Could you check a few things on this model? Use its own coordinates, in mm. Face numbers are marked on the shaded views. A direction names the side the tool comes from. Give positions to 0.01 mm unless a question says otherwise; leave off trailing zeros. Write each loop counter-clockwise with the first axis right and the second up, starting at its lowest first coordinate (ties: lowest second). Pieces come first, ordered by that corner, then holes. Notation, with made-up numbers: (60, -39) - (103, -39) arc R13 cw to (103, -30) - close; hole circle Ø3 at (72.25, 76). An arc over 180 degrees is marked (long way). Answer in a Markdown table with one row per item.
Autodesk Inventor part; units mm, degrees
ref_plane "YZ Plane" through (0, 0, 0) normal (1, 0, 0) x (0, 1, 0)
ref_plane "XZ Plane" through (0, 0, 0) normal (0, 1, 0) x (-1, 0, 0)
ref_plane "XY Plane" through (0, 0, 0) normal (0, 0, 1) x (1, 0, 0)
sketch "スケッチ1" plane through (0, 0, 0) normal (0, 0, 1) x (1, 0, 0)
  circle A0 centre (5, 5) radius 1.55
  circle A1 centre (5, -5) radius 1.55
  line L0 (0, 0) -> (60, 0) construction
  circle A2 centre (60, 0) radius 1.55
  line L1 (0, 10) -> (0, -10)
  line L2 (0, -10) -> (10, -10)
  line L3 (10, -10) -> (60.4762, -5.9811)
  line L4 (10, 10) -> (60.4762, 5.9811)
  arc A3 (60.4762, -5.9811) -> (60.4762, 5.9811) centre (60, 0) ccw
  line L5 (55.0583, -3.4029) -> (11, -6.9109)
  line L6 (55.0583, 3.4029) -> (11, 6.9109)
  arc A4 (55.0583, 3.4029) -> (55.0583, -3.4029) centre (60, 0) ccw
  line L7 (11, -6.9109) -> (11, 6.9109)
  line L8 (5, -5) -> (5, 5) construction
  line L9 (0, 10) -> (10, 10)
  line L10 (8.01, 6.7378) -> (8.01, 3.2622) construction
  line L11 (8.01, 3.2622) -> (5, 1.5244) construction
  line L12 (5, 1.5244) -> (1.99, 3.2622) construction
  line L13 (1.99, 3.2622) -> (1.99, 6.7378) construction
  line L14 (1.99, 6.7378) -> (5, 8.4756) construction
  line L15 (5, 8.4756) -> (8.01, 6.7378) construction
  arc A5 (4.0907, 2.0494) -> (5.9093, 2.0494) centre (5, 2.5744) ccw construction
  arc A6 (7.1007, 2.7372) -> (8.01, 4.3122) centre (7.1007, 3.7872) ccw construction
  arc A7 (8.01, 5.6878) -> (7.1007, 7.2628) centre (7.1007, 6.2128) ccw construction
  arc A8 (5.9093, 7.9506) -> (4.0907, 7.9506) centre (5, 7.4256) ccw construction
  arc A9 (2.8993, 7.2628) -> (1.99, 5.6878) centre (2.8993, 6.2128) ccw construction
  arc A10 (1.99, 4.3122) -> (2.8993, 2.7372) centre (2.8993, 3.7872) ccw construction
  line L16 (8.01, -6.7378) -> (8.01, -3.2622) construction
  line L17 (8.01, -3.2622) -> (5, -1.5244) construction
  line L18 (5, -1.5244) -> (1.99, -3.2622) construction
  line L19 (1.99, -3.2622) -> (1.99, -6.7378) construction
  line L20 (1.99, -6.7378) -> (5, -8.4756) construction
  line L21 (5, -8.4756) -> (8.01, -6.7378) construction
  arc A11 (5.9093, -2.0494) -> (4.0907, -2.0494) centre (5, -2.5744) ccw construction
  arc A12 (8.01, -4.3122) -> (7.1007, -2.7372) centre (7.1007, -3.7872) ccw construction
  arc A13 (7.1007, -7.2628) -> (8.01, -5.6878) centre (7.1007, -6.2128) ccw construction
  arc A14 (4.0907, -7.9506) -> (5.9093, -7.9506) centre (5, -7.4256) ccw construction
  arc A15 (1.99, -5.6878) -> (2.8993, -7.2628) centre (2.8993, -6.2128) ccw construction
  arc A16 (2.8993, -2.7372) -> (1.99, -4.3122) centre (2.8993, -3.7872) ccw construction
  circle A17 centre (60, 0) radius 1.55
  line L22 (63.51, 2.0265) -> (63.51, -2.0265)
  line L23 (63.51, -2.0265) -> (60, -4.053)
  line L24 (60, -4.053) -> (56.49, -2.0265)
  line L25 (56.49, -2.0265) -> (56.49, 2.0265)
  line L26 (56.49, 2.0265) -> (60, 4.053)
  line L27 (60, 4.053) -> (63.51, 2.0265)
  arc A18 (59.0907, -3.528) -> (60.9093, -3.528) centre (60, -3.003) ccw
  arc A19 (62.6007, -2.5515) -> (63.51, -0.9765) centre (62.6007, -1.5015) ccw
  arc A20 (63.51, 0.9765) -> (62.6007, 2.5515) centre (62.6007, 1.5015) ccw
  arc A21 (60.9093, 3.528) -> (59.0907, 3.528) centre (60, 3.003) ccw
  arc A22 (57.3993, 2.5515) -> (56.49, 0.9765) centre (57.3993, 1.5015) ccw
  arc A23 (56.49, -0.9765) -> (57.3993, -2.5515) centre (57.3993, -1.5015) ccw
  line L28 (60, 4.053) -> (60, -4.053) construction
  circle A24 centre (5, 5) radius 3.005
  circle A25 centre (5, -5) radius 3.005
  point P0 (5, 0)
  point P1 (8.01, 3.2622)
  point P2 (8.01, 6.7378)
  point P3 (5, 8.4756)
  point P4 (1.99, 6.7378)
  point P5 (2.8993, 2.7372)
  point P6 (1.99, 4.3122)
  point P7 (1.99, 5.6878)
  point P8 (2.8993, 7.2628)
  point P9 (4.0907, 7.9506)
  point P10 (5.9093, 7.9506)
  point P11 (7.1007, 7.2628)
  point P12 (8.01, 5.6878)
  point P13 (8.01, 4.3122)
  point P14 (7.1007, 2.7372)
  point P15 (7.1007, -2.7372)
  point P16 (8.01, -4.3122)
  point P17 (8.01, -5.6878)
  point P18 (7.1007, -7.2628)
  point P19 (5.9093, -7.9506)
  point P20 (4.0907, -7.9506)
  point P21 (2.8993, -7.2628)
  point P22 (1.99, -5.6878)
  point P23 (1.99, -4.3122)
  point P24 (2.8993, -2.7372)
  point P25 (1.99, -6.7378)
  point P26 (5, -8.4756)
  point P27 (56.49, 2.0265)
  point P28 (56.49, -2.0265)
  point P29 (62.6007, -2.5515)
  point P30 (57.3993, -2.5515)
  point P31 (56.49, -0.9765)
  point P32 (56.49, 0.9765)
  point P33 (57.3993, 2.5515)
  point P34 (59.0907, 3.528)
  point P35 (60.9093, 3.528)
  point P36 (62.6007, 2.5515)
  point P37 (63.51, 0.9765)
  point P38 (63.51, -0.9765)
  dimension "d0" = 10
  dimension "d1" = 3.1
  dimension "d2" = 3.1
  dimension "d3" = 60
  dimension "d4" = 6
  dimension "d33" = 3
  dimension "d34" = 6
  dimension "d35" = 6
  dimension "d40" = 20
  dimension "d41" = 5
  dimension "d42" = 10
  dimension "d43" = 6.02
  dimension "d44" = 2.1
  dimension "d47" = 360
  dimension "d57" = 3.1
  dimension "d58" = 7.02
  dimension "d59" = 2.1
  dimension "d60" = 360
  dimension "d62" = 6.01
extrude "押し出し1" add sketch "スケッチ1" along normal blind 5 contours L9 L4 A3 L3 L2 L1
extrude "押し出し5" add sketch "スケッチ1" along normal blind 3.5 contours A24 | A25
extrude "押し出し6" add sketch "スケッチ1" along normal blind 2 contours A20 L22 | L22 L23 L24 L25 L26 L27 | L27 A20 | A19 L22 | L27 A21 | A19 L23 | L26 A21 | A18 L23 | L26 A22 | A18 L24 | L25 A22 | A23 L24 | L25 A23
extrude "押し出し7" add sketch "スケッチ1" along normal blind 1 contours L5 L7 L6 A4
fillet "フィレット2" radius 2 6 edges at (11, 6.9109, 3) (11, -6.9109, 3) (55.0583, 3.4029, 3) (55.0583, -3.4029, 3) (0, -10, 2.5) (0, 10, 2.5)
properties part number "Trunk_handle_frame" material "アセタール樹脂、黒"
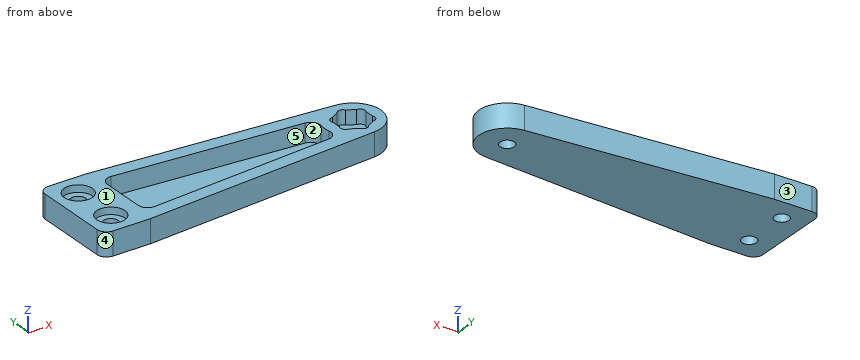
1) On a 3-axis mill with a long thin cutter (end or side, diameter ignored), from which of +Z, -Z, +X, -X, +Y, -Y can I reach the whole of each face in a straight line? I mean the marked faces 1 and 2. Say none if no direction works.
Check values:
| item | result |
|---|---|
| face 1 | +Z, +X, -X, +Y, -Y |
| face 2 | +Z |
2) Imagine slicing it at B-B (y = 0). List the corners of the cut face in (x, z) for me, then the cut area to 3 significant figures.
Check values:
| item | result |
|---|---|
| outline | (0, 0) - (58.45, 0) - (58.45, 2) - (56.49, 2) - (56.49, 5) - (54, 5) - (54, 1) - (11, 1) - (11, 5) - (0, 5) - close; (61.55, 0) - (66, 0) - (66, 5) - (63.51, 5) - (63.51, 2) - (61.55, 2) - close |
| area | 131 mm2 |
3) Imagine slicing it at C-C (z = 4.1). State how many separate pieces and enclosed holes the cut face has, then the cut area to 3 significant figures.
Check values:
| item | result |
|---|---|
| separate pieces | 1 |
| enclosed holes | 4 |
| area | 511 mm2 |
4) Imagine slicing it at D-D (x = 19.5). List the corners of the cut face in (y, z) for me.
Check values:
| item | result |
|---|---|
| outline | (-9.24, 0) - (9.24, 0) - (9.24, 5) - (6.23, 5) - (6.23, 1) - (-6.23, 1) - (-6.23, 5) - (-9.24, 5) - close |
5) We'd pull the mould along X, two halves only. Please class the marked faces 3, 4 and 5: +X half, -X half, draft (parallel to the pull), parting line (faces both ways), or undercut.
Check values:
| item | result |
|---|---|
| face 3 | draft |
| face 4 | -X half |
| face 5 | undercut |
6) Will this pin go through, and if not, where does the flat tip stop? P1, Ø3, axis at x = 5, y = -6, coming from the +Z side.
Check values:
| item | result |
|---|---|
| P1 | stops at z = 3.5 |
7) If I drill on line 1 (Y direction, x = 5, z = 4.7) (3 decimals); line 2 (Y direction, x = 5, z = 0.75); line 3 (X direction, y = -0.5, z = 3.65), over which ranges is the centre line in solid material (lowest first)?
Check values:
| item | result |
|---|---|
| line 1 | y = -10 to -8.005, -1.995 to 1.995, 8.005 to 10 |
| line 2 | y = -10 to -6.55, -3.45 to 3.45, 6.55 to 10 |
| line 3 | x = 0 to 11, 54.02 to 56.49, 63.51 to 65.98 |
8) Imagine slicing it at A-A (x = 5). List the corners of the cut face in (y, z) for me (3 decimals), then the cut area to 3 significant figures.
Check values:
| item | result |
|---|---|
| outline | (-10, 0) - (-6.55, 0) - (-6.55, 3.5) - (-8.005, 3.5) - (-8.005, 5) - (-10, 5) - close; (-3.45, 0) - (3.45, 0) - (3.45, 3.5) - (1.995, 3.5) - (1.995, 5) - (-1.995, 5) - (-1.995, 3.5) - (-3.45, 3.5) - close; (6.55, 0) - (10, 0) - (10, 5) - (8.005, 5) - (8.005, 3.5) - (6.55, 3.5) - close |
| area | 60.3 mm2 |
